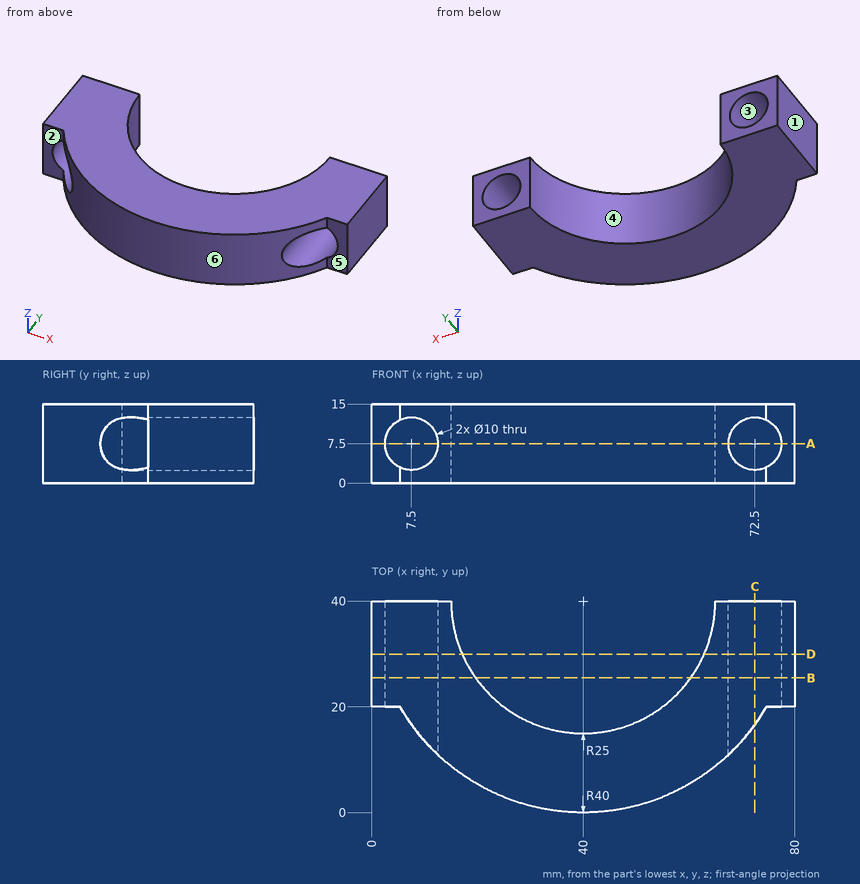
Part print with two shaded views. Sizes in mm from the minimum x, y, z corner. A direction names the side the tool comes from. Coordinates: 2 decimals unless noted, no trailing zeros. Write each loop counter-clockwise with the first axis right and the second up, starting at its lowest first coordinate (ties: lowest second). Pieces come first, ordered by that corner, then holes. Notation, with made-up numbers: (23.5, 55) - (36.5, 55) arc R18 cw to (36.5, 62) - close; hole circle Ø7 at (-27, 59.5). An arc over 180 degrees is marked (long way). Put each result on its own line as item: value.
1. Band-saw the part on C-C (x = 72.5). Write the cut outline in (y, z), then the cut area to 3 significant figures.
Final values:
outline: (16.68, 0) - (40, 0) - (40, 2.5) - (16.68, 2.5) - close; (16.68, 12.5) - (40, 12.5) - (40, 15) - (16.68, 15) - close
area: 117 mm²
2. Band-saw the part on A-A (z = 7.5). Write the cut outline in (x, y).
Final values:
outline: (0, 20) - (2.5, 20) - (2.5, 40) - (0, 40) - close; (12.5, 10.95) arc R40 ccw to (67.5, 10.95) - (67.5, 40) - (65, 40) arc R25 cw to (15, 40) - (12.5, 40) - close; (77.5, 20) - (80, 20) - (80, 40) - (77.5, 40) - close
3. Band-saw the part on B-B (y = 25.5). Write the cut outline in (x, z).
Final values:
outline: (0, 0) - (19.63, 0) - (19.63, 15) - (0, 15) - close; (60.37, 0) - (80, 0) - (80, 15) - (60.37, 15) - close; hole circle Ø10 at (7.5, 7.5); hole circle Ø10 at (72.5, 7.5)
4. Probe line 1 along X through (y, z) = (26, 11.25); line 2 along X through (y, z) = (23.5, 9.25); line 3 along Z through (x, y) = (7.5, 21.5). List the from-to ranges inside material, lowest first. Write a range as [from, to].
Final values:
line 1: x = [0, 4.19], [10.81, 19.29], [60.71, 69.19], [75.81, 80]
line 2: x = [0, 2.82], [12.18, 21.22], [58.78, 67.82], [77.18, 80]
line 3: z = [0, 2.5], [12.5, 15]
5. Band-saw the part on D-D (y = 30). Write the cut outline in (x, z), then the cut area to 3 significant figures.
Final values:
outline: (0, 0) - (17.09, 0) - (17.09, 15) - (0, 15) - close; (62.91, 0) - (80, 0) - (80, 15) - (62.91, 15) - close; hole circle Ø10 at (7.5, 7.5); hole circle Ø10 at (72.5, 7.5)
area: 356 mm²
6. Two-plate mould, pull along X, no slides. Class the marked faces 3, 4, 5 and 6: +X half, -X half, draft (parallel to the pull), parting line (faces both ways), or undercut.
Final values:
face 3: undercut
face 4: undercut
face 5: draft
face 6: parting line
7. 3-axis set-ups, long thin cutter, end or side, ignore diameter. For the marked faces 1 and 2: which of +Z, -Z, +X, -X, +Y, -Y reach the whole face in a straight line?
Final values:
face 1: +Z, -Z, -X, +Y, -Y
face 2: +Z, -Z, -X, -Y
8. Flat gauge pins, fed straight in: pin 1 Ø8 at (x, z) = (72.5, 7.5) entering from +Y; pin 2 Ø2 at (x, z) = (27, 13) entering from +Y; pin 3 Ø1 at (x, z) = (21.5, 5.5) entering from -Y; pin 4 Ø3 at (x, z) = (20, 11) entering from +Y. Where does each tip first touch, or does it go through?
Final values:
pin 1: passes through
pin 2: stops at y = 19.29
pin 3: stops at y = 4.28
pin 4: stops at y = 27.24
